Verification items for the finished model (mm, model axes). A direction names the side the tool comes from. Give positions to 0.01 mm unless a question says otherwise; leave off trailing zeros. Loops run counter-clockwise (first coordinate to the right, second up) from the corner with the lowest first, then second, coordinate; pieces in that order, holes last. Notation, with made-up numbers: M 53.25,-16.5 L 93.25,-16.5 A15 ccw 93.25,-3.5 Z; hole C 50,-21 d6. An arc over 180 degrees is marked long. Use a Markdown table: item, result.
from build123d import *

# Parameters (mm, degrees)
ESQUISSE2_R                  = 1.5
ENL_V_MAT_EXTRU_1_DEPTH      = 86.23333422
ESQUISSE4_R                  = 1.5
ENL_V_MAT_EXTRU_2_DEPTH      = 86.23333422
R_P_TITION_CIRCULAIRE1_COUNT = 3
ESQUISSE5_R                  = 0.75
ENL_V_MAT_EXTRU_3_DEPTH      = 86.23333422


with BuildPart() as part:
    # Esquisse1 → Base-Révolution (revolve)
    with BuildSketch(Plane(origin=(0, 0, 0), x_dir=(0, 0, -1), z_dir=(1, 0, 0)), mode=Mode.PRIVATE) as base_r_volution_sk:
        with BuildLine():
            Line((0, 41.875), (0, 35))
            Line((0, 35), (10, 35))
            Line((10, 35), (10, 33.25))
            Line((10, 33.25), (20.3, 33.25))
            ThreePointArc((20.3, 33.25), (41.210897279, 31.167034961), (61.3, 25))
            Line((61.3, 25), (61.3, 25.5))
            ThreePointArc((61.3, 25.5), (41.215843277, 31.704165587), (20.3, 33.8))
            Line((20.3, 33.8), (11, 33.8))
            Line((11, 33.8), (11, 36))
            Line((11, 36), (1, 36))
            Line((1, 36), (1, 41.875))
            Line((1, 41.875), (0, 41.875))
        make_face()
    revolve(base_r_volution_sk.sketch.rotate(Axis((0, 0, 48.008611825), (0, 0, -1)), 90), axis=Axis((0, 0, 48.008611825), (0, 0, -1)))

    # Esquisse2 → Enlèv. mat.-Extru.1 (cut, through all)
    with BuildSketch(Plane.XY):
        with Locations((0, -37.995)):
            Circle(ESQUISSE2_R)
        with Locations((0, 38)):
            Circle(ESQUISSE2_R)
        with Locations((-18.9975, -32.904635217)):
            Circle(ESQUISSE2_R)
        with Locations((-37.995, 0)):
            Circle(ESQUISSE2_R)
        with Locations((-32.904635217, 18.9975)):
            Circle(ESQUISSE2_R)
        with Locations((-18.9975, 32.904635217)):
            Circle(ESQUISSE2_R)
        with Locations((18.9975, 32.904635217)):
            Circle(ESQUISSE2_R)
        with Locations((32.904635217, 18.9975)):
            Circle(ESQUISSE2_R)
        with Locations((37.995, 0)):
            Circle(ESQUISSE2_R)
        with Locations((18.9975, -32.904635217)):
            Circle(ESQUISSE2_R)
        with Locations((32.908965344, -19)):
            Circle(ESQUISSE2_R)
        with Locations((-32.908965344, -19)):
            Circle(ESQUISSE2_R)
    extrude(amount=-ENL_V_MAT_EXTRU_1_DEPTH, mode=Mode.SUBTRACT)

    # Esquisse4 → Enlèv. mat.-Extru.2 (cut, through all)
    with BuildSketch(Plane(origin=(0, 0, 0), x_dir=(1, 0, 0), z_dir=(0, 1, 0))):
        with Locations(Location((0, 9, 0), (0, 0, 270))):
            Circle(ESQUISSE4_R)
    enl_v_mat_extru_2 = extrude(amount=-ENL_V_MAT_EXTRU_2_DEPTH, mode=Mode.SUBTRACT)

    # Répétition circulaire1: Enlèv. mat.-Extru.2 ×3 about axis
    r_p_tition_circulaire1_axis = Axis((0, 0, 48.008611825), (0, 0, -1))
    for i in range(1, R_P_TITION_CIRCULAIRE1_COUNT):
        add(enl_v_mat_extru_2.rotate(r_p_tition_circulaire1_axis, i * 360 / R_P_TITION_CIRCULAIRE1_COUNT), mode=Mode.SUBTRACT)

    # Esquisse5 → Enlèv. mat.-Extru.3 (cut, through all)
    with BuildSketch(Plane(origin=(0, 0, 0), x_dir=(0, 0, -1), z_dir=(0, 1, 0))):
        with Locations(Location((55.8, 0, 0), (0, 0, 30.651170267))):
            Circle(ESQUISSE5_R)
    extrude(amount=ENL_V_MAT_EXTRU_3_DEPTH, mode=Mode.SUBTRACT)


solid = part.part
(1) Set-up check for faces 4 (the cylindrical face through (17.87, -28.04, -15.22)), 5 (the cylindrical face through (0.07, -34.9, -10.5)), 6 (the cylindrical face through (-0.325, 36.536, -0.493)): record each of +Z, -Z, +X, -X, +Y, -Y from which the full face is reachable in a straight line by a thin tool's end or side.
Results below:
| item | result |
|---|---|
| face 4 | +Z |
| face 5 | -Y |
| face 6 | +Z, -Z |
(2) Material ranges on line 1 (Y direction, x = 0, z = -0.3) (3 decimals); line 2 (Y direction, x = 0, z = -17); line 3 (X direction, y = -27, z = -47), recorded low to high.
Results below:
| item | result |
|---|---|
| line 1 | -41.875 to -39.495, -36.495 to -35, 35 to 36.5, 39.5 to 41.875 |
| line 2 | -33.8 to -33.25, 33.25 to 33.8 |
| line 3 | -13.89 to -12.69, 12.69 to 13.89 |
(3) Cross-section at B-B on y = 38. Record the cut outline in (x, z), then the cut area to 3 significant figures.
Results below:
| item | result |
|---|---|
| outline | M -17.59,-1 L -1.5,-1 L -1.5,0 L -17.59,0 Z; M 1.5,-1 L 17.59,-1 L 17.59,0 L 1.5,0 Z |
| area | 32.2 mm^2 |
(4) Cross-section at C-C on z = -17. Record the cut outline in (x, y).
Results below:
| item | result |
|---|---|
| outline | C 0,0 d67.6; hole C 0,0 d66.5 |
(5) Draft check along X on faces 1 (the flat face through (-16.9, 18.8, -61.3)), 2 (the flat face through (-31, -13, -10)), 3 (the cylindrical face through (-26.533, -24.331, -5.93)). Enter one of: +X half, -X half, draft (parallel to the pull), parting line (faces both ways), or undercut.
Results below:
| item | result |
|---|---|
| face 1 | draft |
| face 2 | undercut |
| face 3 | parting line |
(6) Gauge pin test, flat ends, axial feed: P1, Ø1.4, axis at x = 0, z = -55.8, coming from the -Y side; P2, Ø10, axis at y = -18, z = -40.5, coming from the -X side; P3, Ø1.5, axis at y = -0.5, z = -23.5, coming from the +X side. Record the tip position at first contact, or that the pin passes through.
Results below:
| item | result |
|---|---|
| P1 | y = -27.89 |
| P2 | x = -29.29 |
| P3 | x = 33.77 |
(7) Cross-section at A-A on y = 0. State how many separate pieces and enclosed holes the cut face has, then the cut area to 3 significant figures.
Results below:
| item | result |
|---|---|
| separate pieces | 4 |
| enclosed holes | 0 |
| area | 85.3 mm^2 |
